Work out the finished part from the listing and answer in its coordinate system (mm). A direction names the side the tool comes from. Round coordinates to 2 decimals unless told otherwise and drop trailing zeros. Loops run counter-clockwise (first coordinate to the right, second up) from the corner with the lowest first, then second, coordinate; pieces in that order, holes last. Notation, with made-up numbers: (25, -39.75) -> (62, -39.75) arc R27 ccw to (62, -6.75) -> close; hole circle Ø7 at (18.25, 58). An arc over 180 degrees is marked (long way). Use one line per item in the form item = value.
```python
from build123d import *

# Parameters (mm, degrees)
SKIZZE1_W                            = 40
SKIZZE1_H                            = 13
AUFSATZ_LINEAR_AUSTRAGEN1_DEPTH      = 10
SKIZZE3_W                            = 40
SKIZZE3_H                            = 7.4
AUFSATZ_LINEAR_AUSTRAGEN3_DEPTH      = 150
SCHNITT_LINEAR_AUSTRAGEN1_DEPTH      = 166.090157187
SCHNITT_LINEAR_AUSTRAGEN1_DEPTH_BACK = 11
SKIZZE4_R                            = 15
SKIZZE7_R                            = 20
AUFSATZ_LINEAR_AUSTRAGEN4_DEPTH      = 0.5
SKIZZE5_R                            = 2.55
SCHNITT_LINEAR_AUSTRAGEN2_DEPTH      = 150
SCHNITT_LINEAR_START                 = -0.5
SKIZZE8_R                            = 15
SCHNITT_LINEAR_AUSTRAGEN4_DEPTH      = 0.5
SKIZZE10_R                           = 2.5
SCHNITT_LINEAR_AUSTRAGEN5_DEPTH      = 17
SKIZZE15_R                           = 4.25
SCHNITT_LINEAR_AUSTRAGEN7_DEPTH      = 5
SKIZZE16_W                           = 10
SKIZZE16_H                           = 10
AUFSATZ_LINEAR_AUSTRAGEN5_DEPTH      = 5.5
SKIZZE17_R                           = 2.5
SCHNITT_LINEAR_AUSTRAGEN8_DEPTH      = 21.6
SKIZZE18_R                           = 4.25
SCHNITT_LINEAR_AUSTRAGEN9_DEPTH      = 4.9


with BuildPart() as part:
    # Skizze1 → Aufsatz-Linear austragen1 (new body)
    with BuildSketch(Plane.XY):
        with Locations((20, 6.5)):
            Rectangle(SKIZZE1_W, SKIZZE1_H)
    extrude(amount=AUFSATZ_LINEAR_AUSTRAGEN1_DEPTH)

    # Skizze3 → Aufsatz-Linear austragen3 (add)
    with BuildSketch(Plane.XY.offset(10)):
        with Locations((20, 9.3)):
            Rectangle(SKIZZE3_W, SKIZZE3_H)
    extrude(amount=AUFSATZ_LINEAR_AUSTRAGEN3_DEPTH)

    # Skizze4 → Schnitt-Linear austragen1 (cut, two sides: drawn at the far end of the back side and taken through both)
    with BuildSketch(Plane.XZ.offset(-5.6).offset(-SCHNITT_LINEAR_AUSTRAGEN1_DEPTH_BACK)):
        with Locations(Location((20, 70, 0), (0, 0, 90))):
            Circle(SKIZZE4_R)
    extrude(amount=SCHNITT_LINEAR_AUSTRAGEN1_DEPTH + SCHNITT_LINEAR_AUSTRAGEN1_DEPTH_BACK, mode=Mode.SUBTRACT)

    # Skizze7 → Aufsatz-Linear austragen4 (add)
    with BuildSketch(Plane.XZ.offset(-5.6)):
        with Locations(Location((20, 70, 0), (0, 0, 180))):
            Circle(SKIZZE7_R)
    extrude(amount=AUFSATZ_LINEAR_AUSTRAGEN4_DEPTH)

    # Skizze5 → Schnitt-Linear austragen2 (cut)
    with BuildSketch(Plane(origin=(0, 5.6, 0), x_dir=(-1, 0, 0), z_dir=(0, -1, 0))):
        with Locations(Location((-20, -130, 0), (0, 0, 90))):
            Circle(SKIZZE5_R)
    extrude(amount=-SCHNITT_LINEAR_AUSTRAGEN2_DEPTH, mode=Mode.SUBTRACT)

    # Skizze8 → Schnitt-Linear austragen4 (cut)
    with BuildSketch(Plane(origin=(0, 5.6, 0), x_dir=(1, 0, 0), z_dir=(0, 1, 0)).offset(SCHNITT_LINEAR_START)):
        with Locations(Location((20, -70, 0), (0, 0, 270))):
            Circle(SKIZZE8_R)
    extrude(amount=SCHNITT_LINEAR_AUSTRAGEN4_DEPTH, mode=Mode.SUBTRACT)

    # Skizze10 → Schnitt-Linear austragen5 (cut)
    with BuildSketch(Plane.XZ):
        with Locations(Location((7.5, 5, 0), (0, 0, 270))):
            Circle(SKIZZE10_R)
        with Locations(Location((32.5, 5, 0), (0, 0, 270))):
            Circle(SKIZZE10_R)
    extrude(amount=-SCHNITT_LINEAR_AUSTRAGEN5_DEPTH, mode=Mode.SUBTRACT)

    # Skizze15 → Schnitt-Linear austragen7 (cut)
    with BuildSketch(Plane(origin=(0, 13, 0), x_dir=(1, 0, 0), z_dir=(0, 1, 0))):
        with Locations(Location((7.5, -5, 0), (0, 0, 270))):
            Circle(SKIZZE15_R)
        with Locations(Location((32.5, -5, 0), (0, 0, 270))):
            Circle(SKIZZE15_R)
    extrude(amount=-SCHNITT_LINEAR_AUSTRAGEN7_DEPTH, mode=Mode.SUBTRACT)

    # Skizze16 → Aufsatz-Linear austragen5 (add)
    with BuildSketch(Plane.XZ.offset(-5.6)):
        with Locations((5, 155)):
            Rectangle(SKIZZE16_W, SKIZZE16_H)
        with Locations((35, 155)):
            Rectangle(SKIZZE16_W, SKIZZE16_H)
    extrude(amount=AUFSATZ_LINEAR_AUSTRAGEN5_DEPTH)

    # Skizze17 → Schnitt-Linear austragen8 (cut)
    with BuildSketch(Plane(origin=(0, 13, 0), x_dir=(1, 0, 0), z_dir=(0, 1, 0))):
        with Locations(Location((5, -155.5, 0), (0, 0, 270))):
            Circle(SKIZZE17_R)
        with Locations(Location((35, -155.5, 0), (0, 0, 270))):
            Circle(SKIZZE17_R)
    extrude(amount=-SCHNITT_LINEAR_AUSTRAGEN8_DEPTH, mode=Mode.SUBTRACT)

    # Skizze18 → Schnitt-Linear austragen9 (cut)
    with BuildSketch(Plane(origin=(0, 13, 0), x_dir=(1, 0, 0), z_dir=(0, 1, 0))):
        with Locations(Location((5, -155.5, 0), (0, 0, 270))):
            Circle(SKIZZE18_R)
        with Locations(Location((35, -155.5, 0), (0, 0, 270))):
            Circle(SKIZZE18_R)
    extrude(amount=-SCHNITT_LINEAR_AUSTRAGEN9_DEPTH, mode=Mode.SUBTRACT)


solid = part.part
```
(1) For a pull along Z with two mould halves and no side action, classify faces 6 (the cylindrical face through (28.35, 10.54, 4.08)), 7 (the flat face through (34.9, 0.1, 152.8)), 8 (the flat face through (20, 7, 0)), 9 (the flat face through (20, 8, 160)) as +Z half, -Z half, draft (parallel to the pull), parting line (faces both ways), or undercut.
Completed:
face_6 = undercut
face_7 = draft
face_8 = -Z half
face_9 = +Z half
(2) Find section D-D, the plane z = 25.5. Write down the section's boundary in (x, y), then the cut area to 3 significant figures.
Completed:
outline = (0, 5.6) -> (40, 5.6) -> (40, 13) -> (0, 13) -> close
area = 296 mm2
(3) Given P1, Ø12, axis at x = 35.5, z = 103.5, coming from the -Y side; P2, Ø7, axis at x = 5, z = 155.5, coming from the -Y side; P3, Ø5, axis at y = 7, z = 62, coming from the -X side; P4, Ø2.5, axis at x = 9, z = 7, coming from the +Y side, each flat-ended and moving along its own axis, determine where each tip first touches the part or whether it passes through.
Completed:
P1 = 5.6
P2 = 0.1
P3 = 0
P4 = 8
(4) Find section C-C, the plane x = 20. Write down the section's boundary in (y, z).
Completed:
outline = (0, 0) -> (13, 0) -> (13, 55) -> (5.1, 55) -> (5.1, 50) -> (5.6, 50) -> (5.6, 10) -> (0, 10) -> close; (5.1, 85) -> (13, 85) -> (13, 127.45) -> (5.6, 127.45) -> (5.6, 90) -> (5.1, 90) -> close; (5.6, 132.55) -> (13, 132.55) -> (13, 160) -> (5.6, 160) -> close
(5) Consider L1, parallel to X at y = 10, z = 5; L2, parallel to X at y = 9.15, z = 155.5; L3, parallel to X at y = 9, z = 70. Determine where each line is inside the solid, lowest interval first.
Completed:
L1 = 0 to 3.25, 11.75 to 28.25, 36.75 to 40
L2 = 0 to 0.75, 9.25 to 30.75, 39.25 to 40
L3 = 0 to 5, 35 to 40
(6) Find section A-A, the plane y = 3. Write down the section's boundary in (x, z), then the cut area to 3 significant figures.
Completed:
outline = (0, 0) -> (40, 0) -> (40, 10) -> (0, 10) -> close; (0, 150) -> (10, 150) -> (10, 160) -> (0, 160) -> close; (30, 150) -> (40, 150) -> (40, 160) -> (30, 160) -> close; hole circle Ø5 at (5, 155.5); hole circle Ø5 at (7.5, 5); hole circle Ø5 at (32.5, 5); hole circle Ø5 at (35, 155.5)
area = 521 mm2
(7) Find section B-B, the plane z = 5. Write down the section's boundary in (x, y).
Completed:
outline = (0, 0) -> (5, 0) -> (5, 8) -> (3.25, 8) -> (3.25, 13) -> (0, 13) -> close; (10, 0) -> (30, 0) -> (30, 8) -> (28.25, 8) -> (28.25, 13) -> (11.75, 13) -> (11.75, 8) -> (10, 8) -> close; (35, 0) -> (40, 0) -> (40, 13) -> (36.75, 13) -> (36.75, 8) -> (35, 8) -> close
(8) For faces 1 (the flat face through (10, 3, 155)), 2 (the cylindrical face through (20.77, 9.25, 127.57)), 3 (the flat face through (35.1, 8.1, 158.3)), 4 (the flat face through (5, 3, 150)), 5 (the flat face through (0, 9, 79)), determine the directions among +Z, -Z, +X, -X, +Y, -Y from which every point of the face is accessible in a straight line to the end or side of a thin tool.
Completed:
face_1 = +Z, -Y
face_2 = +Y, -Y
face_3 = +Y
face_4 = +X, -X, -Y
face_5 = +Z, -Z, -X, +Y, -Y
